```python
from build123d import *

# Parameters (mm, degrees)
F0_R      = 50
F1_DEPTH  = 15
F2_R      = 32.5
F3_DEPTH  = 5
F4_R      = 27.5
F5_DEPTH  = 21
F6_R      = 26
F7_DEPTH  = 2
F8_R      = 27.5
F9_DEPTH  = 44
F10_R     = 26
F11_DEPTH = 2
F12_R     = 27.5
F13_DEPTH = 21
F14_R     = 10
F15_DEPTH = 34
F17_D     = 8.5
F19_D     = 8.5
F19_DEPTH = 27
F19_TIP   = 2.5536576309
F20_SIZE  = 2
F21_SIZE  = 0.5
F22_SIZE  = 0.5


with BuildPart() as f1:
    # F0 (on Top) → F1 (new body)
    with BuildSketch(Plane.XY):
        Circle(F0_R)
    extrude(amount=F1_DEPTH)

    # F2 (on face) → F3 (join)
    with BuildSketch(Plane.XY.offset(15)):
        Circle(F2_R)
    extrude(amount=F3_DEPTH)

    # F4 (on face) → F5 (join)
    with BuildSketch(Plane.XY.offset(20)):
        Circle(F4_R)
    extrude(amount=F5_DEPTH)

    # F6 (on face) → F7 (join)
    with BuildSketch(Plane.XY.offset(41)):
        Circle(F6_R)
    extrude(amount=F7_DEPTH)

    # F8 (on face) → F9 (join)
    with BuildSketch(Plane.XY.offset(43)):
        Circle(F8_R)
    extrude(amount=F9_DEPTH)

    # F10 (on face) → F11 (join)
    with BuildSketch(Plane.XY.offset(87)):
        Circle(F10_R)
    extrude(amount=F11_DEPTH)

    # F12 (on face) → F13 (join)
    with BuildSketch(Plane.XY.offset(89)):
        Circle(F12_R)
    extrude(amount=F13_DEPTH)

    # F14 (on face) → F15 (join)
    with BuildSketch(Plane.XY.offset(110)):
        Circle(F14_R)
    extrude(amount=F15_DEPTH)

    # F17 (through all)
    with Locations(Plane(origin=(0, 0, 0), x_dir=(1, 0, 0), z_dir=(0, 0, -1))):
        with Locations((0, 42), (42, 0), (0, -42), (-42, 0)):
            Hole(F17_D / 2)

    # F19
    with Locations(Plane.XY.offset(110)):
        with Locations((0, 20), (20, 0), (0, -20), (-20, 0)):
            Hole(F19_D / 2, depth=F19_DEPTH)
            with Locations((0, 0, -(F19_DEPTH + F19_TIP / 2))):  # 118° drill point
                Cone(0, F19_D / 2, F19_TIP, mode=Mode.SUBTRACT)

    # F20
    f20_edges = [f1.edges().sort_by_distance(p)[0] for p in [
        (-50, 0, 0),
    ]]
    chamfer(f20_edges, length=F20_SIZE)

    # F21
    f21_edges = [f1.edges().sort_by_distance(p)[0] for p in [
        (-32.5, 0, 20),
    ]]
    chamfer(f21_edges, length=F21_SIZE)

    # F22
    f22_edges = [f1.edges().sort_by_distance(p)[0] for p in [
        (-27.5, 0, 110),
    ]]
    chamfer(f22_edges, length=F22_SIZE)


solid = f1.part
```
Source: CAD feature listing. Evaluate the final solid. Frame: model axes, mm. A direction names the side the tool comes from. Round coordinates to 2 decimals unless told otherwise and drop trailing zeros. Use CSV: the item, a comma, the result in double quotes. Start each with the question number.
Q1. Pull-direction query (Z, two-part tool) for faces 1 (the face through (10.1, -24.3, 87)), 2 (the face through (3.37, -39.41, 7.6)), 3 (the face through (-1, -33, 15)); classes: +Z half, -Z half, draft (parallel to the pull), parting line (faces both ways), or undercut.
Q2. Line query: line 1 (Y direction, x = 0, z = 31); line 2 (Z direction, x = 23, y = 20); line 3 (Z direction, x = 38, y = -28.5). Output: solid intervals per line, ascending. Write a range as from..to.
Q3. Access query for faces 4 (the face through (10.1, -24.3, 43)), 5 (the face through (46.246, -0.187, 7.605)), 6 (the face through (-16.868, 2.872, 96.311)). Directions: +Z, -Z, +X, -X, +Y, -Y. A direction counts if a zero-diameter tool reaches every point of the face in a straight line with its end or side. Return the directions, or none.
Q4. First-contact query: P1, Ø6, axis at y = 5, z = 61.5, coming from the +X side; P2, Ø6, axis at y = 6, z = 108, coming from the +X side; P3, Ø8, axis at x = -26, y = -14.5, coming from the +Z side. Flat tips, straight axial feed; report the tip coordinate or a pass-through.
Results found:
1,face 1,"undercut"
1,face 2,"draft"
1,face 3,"+Z half"
2,line 1,"-27.5..27.5"
2,line 2,"0..20"
2,line 3,"0..15"
3,face 4,"none"
3,face 5,"+Z, -Z"
3,face 6,"+Z"
4,P1,"x = 27.43"
4,P2,"x = 27.34"
4,P3,"z = 110"
